Design review of the part built by this model. Coordinates are the model's own, in mm. A direction names the side the tool comes from. Give positions to 0.01 mm unless a question says otherwise; leave off trailing zeros. Write each loop counter-clockwise with the first axis right and the second up, starting at its lowest first coordinate (ties: lowest second). Pieces come first, ordered by that corner, then holes. Notation, with made-up numbers: M 72.25,63.5 L 113.25,63.5 A31 ccw 113.25,98.5 Z; hole C -1,49 d2. An arc over 180 degrees is marked long. One line per item, written item: value. Start each with the question number.
```python
from build123d import *

# Parameters (mm, degrees)
ESBO_O1_W                = 150
ESBO_O1_H                = 100
RESSALTO_EXTRUS_O2_DEPTH = 6
ESBO_O3_W                = 90
ESBO_O3_H                = 30
CORTE_EXTRUS_O1_DEPTH    = 91.338253249
ESBO_O4_W                = 6
ESBO_O4_H                = 40
RESSALTO_EXTRUS_O4_DEPTH = 6
ESBO_O5_W                = 6
ESBO_O5_H                = 40
RESSALTO_EXTRUS_O5_DEPTH = 6
ESBO_O7_W                = 30
ESBO_O7_H                = 6
RESSALTO_EXTRUS_O7_DEPTH = 6
ESBO_O8_W                = 30
ESBO_O8_H                = 6
RESSALTO_EXTRUS_O8_DEPTH = 6


with BuildPart() as part:
    # Esboço1 → Ressalto-extrusão2 (new body)
    with BuildSketch(Plane.XY):
        Rectangle(ESBO_O1_W, ESBO_O1_H)
    extrude(amount=RESSALTO_EXTRUS_O2_DEPTH)

    # Esboço3 → Corte-extrusão1 (cut, through all)
    with BuildSketch(Plane.XY.offset(6)):
        with Locations((0, -35)):
            Rectangle(ESBO_O3_W, ESBO_O3_H)
    extrude(amount=-CORTE_EXTRUS_O1_DEPTH, mode=Mode.SUBTRACT)

    # Esboço4 → Ressalto-extrusão4 (add)
    with BuildSketch(Plane(origin=(75, 0, 0), x_dir=(0, 0, -1), z_dir=(1, 0, 0))):
        with Locations((-3, 0)):
            Rectangle(ESBO_O4_W, ESBO_O4_H)
    extrude(amount=RESSALTO_EXTRUS_O4_DEPTH)

    # Esboço5 → Ressalto-extrusão5 (add)
    with BuildSketch(Plane.ZY.offset(75)):
        with Locations((3, 0)):
            Rectangle(ESBO_O5_W, ESBO_O5_H)
    extrude(amount=RESSALTO_EXTRUS_O5_DEPTH)

    # Esboço7 → Ressalto-extrusão7 (add)
    with BuildSketch(Plane.XZ.offset(50)):
        with Locations((60, 3)):
            Rectangle(ESBO_O7_W, ESBO_O7_H)
    extrude(amount=RESSALTO_EXTRUS_O7_DEPTH)

    # Esboço8 → Ressalto-extrusão8 (add)
    with BuildSketch(Plane.XZ.offset(50)):
        with Locations((-60, 3)):
            Rectangle(ESBO_O8_W, ESBO_O8_H)
    extrude(amount=RESSALTO_EXTRUS_O8_DEPTH)


solid = part.part
```
Q1. For P1, Ø3, axis at x = 78, z = 2.5, coming from the -Y side; P2, Ø1.5, axis at y = -41, z = 2, coming from the +X side; P3, Ø3, axis at y = 36, z = 4, coming from the -X side, all flat-tipped, find the tip position at first contact; note any pin that passes through.
Q2. Wall thickness on line 1 (X direction, y = -35, z = 1.65); line 2 (Y direction, x = 30.5, z = 1.7); line 3 (X direction, y = 29, z = 1.4): over which ranges is each line inside the solid? List them lowest first. Write a range as from..to.
Q3. Machinability: for faces 5 (the face through (75, 35, 3)), 6 (the face through (-78, 20, 3)), 7 (the face through (45, -38, 3)), 8 (the face through (75, -38, 3)), which of the approach directions +Z, -Z, +X, -X, +Y, -Y give a long, thin tool a straight path to every point of the face, cutting with its end or side? Answer none if there is none.
Q4. Take a section at D-D, the plane y = 29.5. Give the boundary of the cut face in (x, z), then the cut area to 3 significant figures.
Q5. The part is to be moulded in two halves that separate along X. For faces 1 (the face through (-75, -38, 3)), 2 (the face through (-1, -20, 3)), 3 (the face through (-45, -38, 3)), 4 (the face through (-60, -56, 3)), say which applies: pulls with the +X half, pulls with the -X half, needs draft (parallel to the pull), parting line crosses it, or undercut.
Q6. Take a section at B-B, the plane z = 1.6. Give the boundary of the cut face in (x, y), then the cut area to 3 significant figures.
Q7. Take a section at A-A, the plane y = -25. Give the boundary of the cut face in (x, z).
Q8. Take a section at C-C, the plane x = -32.5. Give the boundary of the cut face in (y, z), then the cut area to 3 significant figures.
Results list:
1. P1: stops at y = -20
1. P2: stops at x = 75
1. P3: stops at x = -75
2. line 1: x = -75..-45, 45..75
2. line 2: y = -20..50
2. line 3: x = -75..75
3. face 5: +Z, -Z, +X, +Y
3. face 6: +Z, -Z, -X, +Y
3. face 7: +Z, -Z, -Y
3. face 8: +Z, -Z, +X, -Y
4. outline: M -75,0 L 75,0 L 75,6 L -75,6 Z
4. area: 900 mm^2
5. face 1: pulls with the -X half
5. face 2: undercut
5. face 3: undercut
5. face 4: needs draft
6. outline: M -81,-20 L -75,-20 L -75,-56 L -45,-56 L -45,-20 L 45,-20 L 45,-56 L 75,-56 L 75,-20 L 81,-20 L 81,20 L 75,20 L 75,50 L -75,50 L -75,20 L -81,20 Z
6. area: 13,100 mm^2
7. outline: M -75,0 L -45,0 L -45,6 L -75,6 Z; M 45,0 L 75,0 L 75,6 L 45,6 Z
8. outline: M -20,0 L 50,0 L 50,6 L -20,6 Z
8. area: 420 mm^2
